Part model, mm, in its own coordinate system. Face numbers are marked on the shaded views. A direction names the side the tool comes from. Coordinates: 2 decimals unless noted, no trailing zeros. Write each loop counter-clockwise with the first axis right and the second up, starting at its lowest first coordinate (ties: lowest second). Pieces come first, ordered by that corner, then holes. Notation, with made-up numbers: (2.25, 61.5) -> (12.25, 61.5) arc R15 cw to (12.25, 88.5) -> close; hole circle Ø7 at (6.5, -4.75). An arc over 180 degrees is marked (long way). Write item = value, one per line.
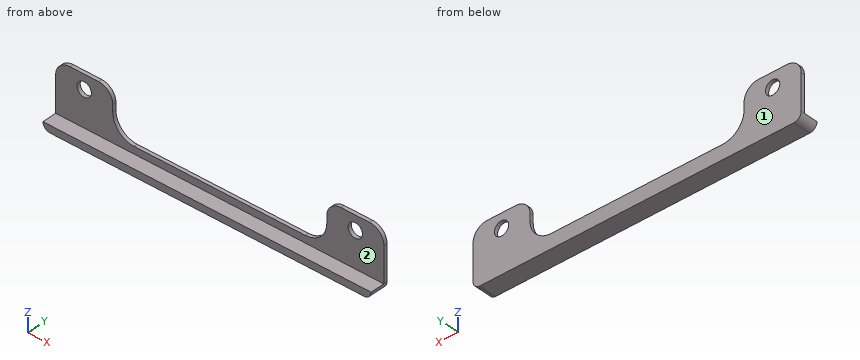
from build123d import *

# Parameters (mm, degrees)
BOSS_EXTRUDE2_DEPTH = 40
SKETCH2_W           = 50
SKETCH2_H           = 35
CUT_EXTRUDE1_DEPTH  = 45
SKETCH3_W           = 50
SKETCH3_H           = 35
CUT_EXTRUDE2_DEPTH  = 45
SKETCH4_W           = 150
SKETCH4_H           = 35
CUT_EXTRUDE3_DEPTH  = 5
CUT_EXTRUDE4_DEPTH  = 50
BOSS_EXTRUDE3_DEPTH = 2.5
BOSS_EXTRUDE4_START = -2.5
BOSS_EXTRUDE4_DEPTH = 2.5
SKETCH10_R          = 7.5
CUT_EXTRUDE5_DEPTH  = 50
CUT_EXTRUDE7_DEPTH  = 10
SKETCH12_W          = 250.559183642
SKETCH12_H          = 50.914019983
CUT_EXTRUDE8_DEPTH  = 10
SKETCH14_R          = 7.5
BOSS_EXTRUDE5_DEPTH = 2.5
SKETCH15_W          = 12.944399718
SKETCH15_H          = 51.5357406
SKETCH15_W_2        = 21.188165756
SKETCH15_H_2        = 60.611007318
CUT_EXTRUDE9_DEPTH  = 50
SKETCH17_W          = 230
SKETCH17_H          = 10
CUT_EXTRUDE10_DEPTH = 50
FILLET3_R           = 5
FILLET4_R           = 10
SKETCH18_R          = 5
CUT_EXTRUDE11_DEPTH = 50


with BuildPart() as part:
    # Sketch1 → Boss-Extrude2 (new body)
    with BuildSketch(Plane(origin=(0, 0, 0), x_dir=(1, 0, 0), z_dir=(0, 1, 0))):
        Polygon((36.951161, 103.273036008), (-88.048839, 103.273036008), (-88.048839, 53.273036008), (-38.048839, 53.273036008), (-38.048839, 93.273036008), (36.951161, 93.273036008), align=None)
        Polygon((161.951161, 103.273036008), (36.951161, 103.273036008), (36.951161, 93.273036008), (111.951161, 93.273036008), (111.951161, 53.273036008), (161.951161, 53.273036008), align=None)
    extrude(amount=-BOSS_EXTRUDE2_DEPTH)

    # Sketch2 → Cut-Extrude1 (cut)
    with BuildSketch(Plane.XY.offset(-53.273036008)):
        with Locations((-63.048839, -20)):
            Rectangle(SKETCH2_W, SKETCH2_H)
    extrude(amount=-CUT_EXTRUDE1_DEPTH, mode=Mode.SUBTRACT)

    # Sketch3 → Cut-Extrude2 (cut)
    with BuildSketch(Plane.XY.offset(-53.273036008)):
        with Locations((136.951161, -20)):
            Rectangle(SKETCH3_W, SKETCH3_H)
    extrude(amount=-CUT_EXTRUDE2_DEPTH, mode=Mode.SUBTRACT)

    # Sketch4 → Cut-Extrude3 (cut)
    with BuildSketch(Plane.XY.offset(-93.273036008)):
        with Locations((36.951161, -20)):
            Rectangle(SKETCH4_W, SKETCH4_H)
    extrude(amount=-CUT_EXTRUDE3_DEPTH, mode=Mode.SUBTRACT)

    # Sketch5 → Cut-Extrude4 (cut)
    with BuildSketch(Plane.XZ.offset(40)):
        with BuildLine():
            ThreePointArc((-80.548839, -103.273036008), (-85.852139859, -101.076336867), (-88.048839, -95.773036008))
            Line((-88.048839, -95.773036008), (-88.048839, -103.273036008))
            Line((-88.048839, -103.273036008), (-80.548839, -103.273036008))
        make_face()
        with BuildLine():
            ThreePointArc((-88.048839, -63.273036008), (-85.119906812, -56.201968196), (-78.048839, -53.273036008))
            Line((-78.048839, -53.273036008), (-88.048839, -53.273036008))
            Line((-88.048839, -53.273036008), (-88.048839, -63.273036008))
        make_face()
        with BuildLine():
            ThreePointArc((-48.048839, -53.273036008), (-40.977771189, -56.201968196), (-38.048839, -63.273036008))
            Line((-38.048839, -63.273036008), (-38.048839, -53.273036008))
            Line((-38.048839, -53.273036008), (-48.048839, -53.273036008))
        make_face()
        with BuildLine():
            Line((111.951161, -53.273036008), (111.951161, -63.273036008))
            ThreePointArc((111.951161, -63.273036008), (114.880093188, -56.201968196), (121.951161, -53.273036008))
            Line((121.951161, -53.273036008), (111.951161, -53.273036008))
        make_face()
        with BuildLine():
            Line((161.951161, -53.273036008), (151.951161, -53.273036008))
            ThreePointArc((151.951161, -53.273036008), (159.022228811, -56.201968196), (161.951161, -63.273036008))
            Line((161.951161, -63.273036008), (161.951161, -53.273036008))
        make_face()
        with BuildLine():
            ThreePointArc((161.951161, -95.773036008), (159.754461858, -101.076336867), (154.451161, -103.273036008))
            Line((154.451161, -103.273036008), (161.951161, -103.273036008))
            Line((161.951161, -103.273036008), (161.951161, -95.773036008))
        make_face()
    extrude(amount=-CUT_EXTRUDE4_DEPTH, mode=Mode.SUBTRACT)

    # Sketch8 → Boss-Extrude3 (add)
    with BuildSketch(Plane.XZ.offset(40)):
        with BuildLine():
            Line((-38.048839, -93.273036008), (-23.048839, -93.273036008))
            ThreePointArc((-23.048839, -93.273036008), (-33.655440718, -88.879637726), (-38.048839, -78.273036008))
            Line((-38.048839, -78.273036008), (-38.048839, -93.273036008))
        make_face()
        with BuildLine():
            ThreePointArc((111.951161, -78.273036008), (107.557762717, -88.879637726), (96.951161, -93.273036008))
            Line((96.951161, -93.273036008), (111.951161, -93.273036008))
            Line((111.951161, -93.273036008), (111.951161, -78.273036008))
        make_face()
    extrude(amount=-BOSS_EXTRUDE3_DEPTH)

    # Sketch9 → Boss-Extrude4 (add)
    with BuildSketch(Plane(origin=(0, 0, 0), x_dir=(1, 0, 0), z_dir=(0, 1, 0)).offset(BOSS_EXTRUDE4_START)):
        with BuildLine():
            Line((111.951161, 93.273036008), (96.951161, 93.273036008))
            ThreePointArc((96.951161, 93.273036008), (107.557762717, 88.879637726), (111.951161, 78.273036008))
            Line((111.951161, 78.273036008), (111.951161, 93.273036008))
        make_face()
        with BuildLine():
            ThreePointArc((-38.048839, 78.273036008), (-33.655440718, 88.879637726), (-23.048839, 93.273036008))
            Line((-23.048839, 93.273036008), (-38.048839, 93.273036008))
            Line((-38.048839, 93.273036008), (-38.048839, 78.273036008))
        make_face()
    extrude(amount=BOSS_EXTRUDE4_DEPTH)

    # Sketch10 → Cut-Extrude5 (cut)
    with BuildSketch(Plane(origin=(0, 0, 0), x_dir=(1, 0, 0), z_dir=(0, 1, 0))):
        with Locations(Location((-62.665129015, 73.273036008, 0), (0, 0, 270))):
            Circle(SKETCH10_R)
        with Locations(Location((136.567451014, 73.273036008, 0), (0, 0, 180))):
            Circle(SKETCH10_R)
    extrude(amount=-CUT_EXTRUDE5_DEPTH, mode=Mode.SUBTRACT)

    # Sketch11 → Cut-Extrude7 (cut)
    with BuildSketch(Plane.XY.offset(-98.273036008)):
        Polygon((161.522228811, -12.5), (-87.619906812, -12.5), (-87.619906812, -16.066465668), (-87.619906812, -37.5), (161.522228811, -37.5), (161.522228811, -16.066465668), align=None)
    extrude(amount=-CUT_EXTRUDE7_DEPTH, mode=Mode.SUBTRACT)


with BuildPart() as cut_extrude7_piece_1:
    # of the separate pieces the step leaves, piece 1, a body of its own (cut_extrude7_pieces)
    add(part.part.solids().sort_by_distance((-80.548839, -12.5, -103.273036008))[0])

    # Sketch14 → Boss-Extrude5 (add)
    with BuildSketch(Plane(origin=(0, 0, 0), x_dir=(1, 0, 0), z_dir=(0, 1, 0))):
        with Locations((-62.665129015, 73.273036008)):
            Circle(SKETCH14_R)
        with Locations((136.567451014, 73.273036008)):
            Circle(SKETCH14_R)
    extrude(amount=-BOSS_EXTRUDE5_DEPTH)

    # Sketch15 → Cut-Extrude9 (cut)
    with BuildSketch(Plane(origin=(0, 0, 0), x_dir=(1, 0, 0), z_dir=(0, 1, 0))):
        with Locations((-84.521038859, 78.400798504)):
            Rectangle(SKETCH15_W, SKETCH15_H)
        with Locations((162.545243878, 78.525177745)):
            Rectangle(SKETCH15_W_2, SKETCH15_H_2)
    extrude(amount=-CUT_EXTRUDE9_DEPTH, mode=Mode.SUBTRACT)

    # Sketch17 → Cut-Extrude10 (cut)
    with BuildSketch(Plane(origin=(0, 0, 0), x_dir=(1, 0, 0), z_dir=(0, 1, 0))):
        with Locations((36.951161, 58.273036008)):
            Rectangle(SKETCH17_W, SKETCH17_H)
    extrude(amount=-CUT_EXTRUDE10_DEPTH, mode=Mode.SUBTRACT)

    # Fillet3
    fillet3_edges = [cut_extrude7_piece_1.edges().sort_by_distance(p)[0] for p in [
        (151.951161, -6.25, -103.273036008),
        (-78.048839, -6.25, -103.273036008),
    ]]
    fillet(fillet3_edges, radius=FILLET3_R - 0.0001)  # a hair under: the kernel refuses the full size

    # Fillet4
    fillet4_edges = [cut_extrude7_piece_1.edges().sort_by_distance(p)[0] for p in [
        (151.951161, -1.25, -63.273036008),
        (-38.048839, -1.25, -63.273036008),
        (111.951161, -1.25, -63.273036008),
        (-78.048839, -1.25, -63.273036008),
    ]]
    fillet(fillet4_edges, radius=FILLET4_R)

    # Sketch18 → Cut-Extrude11 (cut)
    with BuildSketch(Plane.XZ.offset(2.5)):
        with Locations((131.951161, -73.273036008)):
            Circle(SKETCH18_R)
        with Locations((-58.048839, -73.273036008)):
            Circle(SKETCH18_R)
    extrude(amount=-CUT_EXTRUDE11_DEPTH, mode=Mode.SUBTRACT)


with BuildPart() as cut_extrude7_piece_2:
    # of the separate pieces the step leaves, piece 2, a body of its own (cut_extrude7_pieces)
    add(part.part.solids().sort_by_distance((154.451161, -40, -103.273036008))[0])

    # Sketch12 → Cut-Extrude8 (cut)
    with BuildSketch(Plane.XZ.offset(40)):
        with Locations((37.230752821, -78.730046)):
            Rectangle(SKETCH12_W, SKETCH12_H)
    extrude(amount=-CUT_EXTRUDE8_DEPTH, mode=Mode.SUBTRACT)


solid = cut_extrude7_piece_1.part
Q1. Which spindle directions (+Z, -Z, +X, -X, +Y, -Y) get a long thin tool onto all of the face, cutting with end or side? Do the marked faces 1 and 2. Say none if no direction does.
Model answer:
face_1 = +Z, -Z, +X, -X, +Y
face_2 = +Z, +X, -X, -Y
Q2. Saw through at D-D on z = -71. Give the cut face in (x, y), and give its area (3 significant figures).
Model answer:
outline = (-77.79, -2.5) -> (-62.5, -2.5) -> (-62.5, 0) -> (-77.79, 0) -> close; (-53.6, -2.5) -> (-38.31, -2.5) -> (-38.31, 0) -> (-53.6, 0) -> close; (112.21, -2.5) -> (127.5, -2.5) -> (127.5, 0) -> (112.21, 0) -> close; (136.4, -2.5) -> (151.69, -2.5) -> (151.69, 0) -> (136.4, 0) -> close
area = 153 mm²
Q3. Probe line 1 (Z direction, x = 91, y = -9.25); line 2 (Y direction, x = -23.5, z = -95); line 3 (X direction, y = -0.25, z = -76.5). List the from-to ranges inside material, lowest first. Write a range as from..to.
Model answer:
line_1 = -103.27..-98.27
line_2 = -2.5..0
line_3 = -78.05..-61.87, -54.23..-38.05, 111.95..128.13, 135.77..151.95
Q4. Pin check, flat tips, straight feed: pin 1 (6 mm diameter, centred on x = -58.05, z = -73.27, fed in from +Y); pin 2 (5 mm diameter, centred on x = 75, y = -10, fed in from +Z); pin 3 (1.2 mm diameter, centred on x = 15, y = -0.5, fed in from +Z). Stop position of each tip, or through.
Model answer:
pin_1 = through
pin_2 = -98.27
pin_3 = -93.27
Q5. Saw through at C-C on x = 20. Give the cut face in (y, z), and give its area (3 significant figures).
Model answer:
outline = (-12.5, -103.27) -> (0, -103.27) -> (0, -93.27) -> (-2.5, -93.27) -> (-2.5, -98.27) -> (-12.5, -98.27) -> close
area = 75.0 mm²
Q6. Saw through at A-A on z = -86. Give the cut face in (x, y), and give its area (3 significant figures).
Model answer:
outline = (-78.05, -2.5) -> (-35.91, -2.5) -> (-35.91, 0) -> (-78.05, 0) -> close; (109.81, -2.5) -> (151.95, -2.5) -> (151.95, 0) -> (109.81, 0) -> close
area = 211 mm²
